Here's how the part is built. I have some questions about the finished solid (model axes, mm). A direction names the side the tool comes from. Give positions to 0.01 mm unless a question says otherwise; leave off trailing zeros. Order: outer loops, then holes, each group sorted by start corner. A loop starts at its lowest first (then second) coordinate and runs counter-clockwise, first axis right, second up.
from build123d import *

# Parameters (mm, degrees)
CYLINDER_R          = 2
CYLINDER_DEPTH      = 10
CYLINDER_ROLL_ANGLE = 90
BOX004_W            = 10
BOX004_H            = 10
BOX004_DEPTH        = 1
BOX002_W            = 10
BOX002_H            = 10
BOX002_DEPTH        = 1
SKETCH003_R         = 1.15
PAD_DEPTH           = 3
BOX375_W            = 10
BOX375_H            = 10
BOX375_DEPTH        = 1
BOX374_W            = 10
BOX374_H            = 10
BOX374_DEPTH        = 1
SKETCH015_R         = 1.15
PAD001_DEPTH        = 3
SKETCH018_W         = 11
SKETCH018_H         = 23
SKETCH017_W         = 8
SKETCH017_H         = 20
FILLET_R            = 0.2


with BuildPart() as cilindro:
    # Cylinder → Cylinder (new body)
    with BuildSketch(Plane.XY):
        Circle(CYLINDER_R)
    extrude(amount=CYLINDER_DEPTH)


with BuildPart() as cilindro_1:
    # Cylinder roll: moved
    add(cilindro.part.rotate(Axis((0, 0, 0), (1, 0, 0)), CYLINDER_ROLL_ANGLE))


with BuildPart() as cilindro_2:
    # Cylinder placement: moved
    add(cilindro_1.part.moved(Location((-233.5, 0, 6))))


with BuildPart() as cubo004:
    # Box004 → Box004 (new body)
    with BuildSketch(Plane(origin=(-6, 0.7, 0.5), x_dir=(1, 0, 0), z_dir=(0, 0, 1))):
        with Locations((5, 5)):
            Rectangle(BOX004_W, BOX004_H)
    extrude(amount=BOX004_DEPTH)


with BuildPart() as cubo002:
    # Box002 → Box002 (new body)
    with BuildSketch(Plane(origin=(-5, 0.7, -1.5), x_dir=(1, 0, 0), z_dir=(0, 0, 1))):
        with Locations((5, 5)):
            Rectangle(BOX002_W, BOX002_H)
    extrude(amount=BOX002_DEPTH)


with BuildPart() as obj1:
    # Sketch003 → Pad (new body, symmetric)
    with BuildSketch(Plane.XY):
        with BuildLine():
            Line((-0.94599, 5), (0.94599, 5))
            ThreePointArc((2.5, 3.44599), (2.044841, 4.544841), (0.94599, 5))
            Line((2.5, 3.44599), (2.5, 0))
            Line((2.5, 0), (-2.5, 0))
            Line((-2.5, 0), (-2.5, 3.44599))
            ThreePointArc((-0.94599, 5), (-2.044841, 4.544841), (-2.5, 3.44599))
        make_face()
        with Locations((0, 2.97603)):
            Circle(SKETCH003_R, mode=Mode.SUBTRACT)
    extrude(amount=PAD_DEPTH, both=True)

    # Cut004: cut Cubo002
    add(cubo002.part, mode=Mode.SUBTRACT)

    # Cut005: cut Cubo004
    add(cubo004.part, mode=Mode.SUBTRACT)


with BuildPart() as obj1_1:
    # Cut005 placement: moved
    add(obj1.part.moved(Location((-233.5, -6, 0))))


with BuildPart() as cubo374:
    # Box375 → Box375 (new body)
    with BuildSketch(Plane(origin=(-6, 0.7, 0.5), x_dir=(1, 0, 0), z_dir=(0, 0, 1))):
        with Locations((5, 5)):
            Rectangle(BOX375_W, BOX375_H)
    extrude(amount=BOX375_DEPTH)


with BuildPart() as cubo373:
    # Box374 → Box374 (new body)
    with BuildSketch(Plane(origin=(-5, 0.7, -1.5), x_dir=(1, 0, 0), z_dir=(0, 0, 1))):
        with Locations((5, 5)):
            Rectangle(BOX374_W, BOX374_H)
    extrude(amount=BOX374_DEPTH)


with BuildPart() as obj2:
    # Sketch015 → Pad001 (new body, symmetric)
    with BuildSketch(Plane.XY):
        with BuildLine():
            Line((-0.94599, 5), (0.94599, 5))
            ThreePointArc((2.5, 3.44599), (2.044841, 4.544841), (0.94599, 5))
            Line((2.5, 3.44599), (2.5, 0))
            Line((2.5, 0), (-2.5, 0))
            Line((-2.5, 0), (-2.5, 3.44599))
            ThreePointArc((-0.94599, 5), (-2.044841, 4.544841), (-2.5, 3.44599))
        make_face()
        with Locations((0, 2.97603)):
            Circle(SKETCH015_R, mode=Mode.SUBTRACT)
    extrude(amount=PAD001_DEPTH, both=True)

    # Cut103: cut Cubo373
    add(cubo373.part, mode=Mode.SUBTRACT)

    # Cut104: cut Cubo374
    add(cubo374.part, mode=Mode.SUBTRACT)


with BuildPart() as obj2_1:
    # Cut104 placement: moved
    add(obj2.part.moved(Location((-233.5, -6, 12))))


with BuildPart() as obj3:
    # Sketch018 → Loft section 0
    with BuildSketch(Plane(origin=(0, -9, -0.5), x_dir=(1, 0, 0), z_dir=(0, -1, 0))):
        with Locations((-234.807047, 6.068771)):
            Rectangle(SKETCH018_W, SKETCH018_H)
    # Sketch017 → Loft section 1
    with BuildSketch(Plane.XZ.offset(7)):
        with Locations((-234.670651, 5.48801)):
            Rectangle(SKETCH017_W, SKETCH017_H)
    loft()


with BuildPart() as obj3_1:
    # Loft placement: moved
    add(obj3.part.moved(Location((1, 1, 0))))

    # Fusion067: union obj1, obj2
    add(obj1_1.part)
    add(obj2_1.part)

    # Cut105: cut Cilindro
    add(cilindro_2.part, mode=Mode.SUBTRACT)

    # Fillet
    fillet_edges = [obj3_1.edges().sort_by_distance(p)[0] for p in [
        (-235.5, -6, 6),
    ]]
    fillet(fillet_edges, radius=FILLET_R)


solid = obj3_1.part
Q1. If we section it at A-A on y = -5.75: List the corners of the cut face in (x, z) for me.
Filled sheet:
outline: (-236, -3) - (-231, -3) - (-231, 3) - (-236, 3) - close; (-236, 9) - (-231, 9) - (-231, 15) - (-236, 15) - close
Q2. Thinking about a two-plate mould opening in Z: for faces 4 (the face through (-231.44, -1.47, 9.76)), 5 (the face through (-235.498, -7.087, 6.088)), which applies, released by +Z, released by -Z, zero draft, split by the parting line, or undercut?
Filled sheet:
face 4: zero draft
face 5: undercut
Q3. I need wall thicknesses on L1, parallel to Z at x = -232.25, y = -1.25; L2, parallel to Y at x = -233.5, z = -2.25; L3, parallel to Y at x = -234.75, z = 8. Which ranges of each line are inside material? Lowest first, please.
Filled sheet:
L1: z = -3 to -1.5, -0.5 to 0.5, 1.5 to 3, 9 to 10.5, 11.5 to 12.5, 13.5 to 15
L2: y = -8 to -4.17, -1.87 to -1
L3: y = -8 to -6
Q4. For faces 1 (the face through (-233, -5, 9)), 2 (the face through (-236, -5, 0)), 3 (the face through (-234, -1, 2)), which set-ups out of +Z, -Z, +X, -X, +Y, -Y let a thin tool reach every point of the face, with its end or its side?
Filled sheet:
face 1: +X, -X, +Y
face 2: +Z, -Z, -X, +Y
face 3: +Z, -Z, +X, -X, +Y
Q5. If we section it at B-B on x = -233.5: Give the number of separate pieces and of enclosed holes in the cut face, plus the area to 3 significant figures.
Filled sheet:
separate pieces: 8
enclosed holes: 0
area: 59.4 mm2
Q6. I'm going to push flat-ended pins straight in: P1, Ø3.5, axis at x = -233, y = -3, coming from the -Z side; P2, Ø4, axis at y = -2, z = 12, coming from the +X side; P3, Ø3.5, axis at x = -234, y = -3.5, coming from the +Z side. Where does each tip first touch, or does it pass through?
Filled sheet:
P1: stops at z = -3
P2: stops at x = -231
P3: stops at z = 15
